Answer from the drawing. Dimensions are ordinates in mm from the lowest x, y and z of the part. Give positions to 0.01 mm unless a question says otherwise; leave off trailing zeros. Write each loop counter-clockwise with the first axis right and the second up, starting at its lowest first coordinate (ties: lowest second). Pieces come first, ordered by that corner, then holes. Notation, with made-up numbers: (51, 16) - (68, 16) arc R34 cw to (68, 54) - close; hole circle Ø3 at (-23.75, 83.25). An arc over 180 degrees is marked (long way). Answer as a JSON object with one key per item and string values. Group by question number.
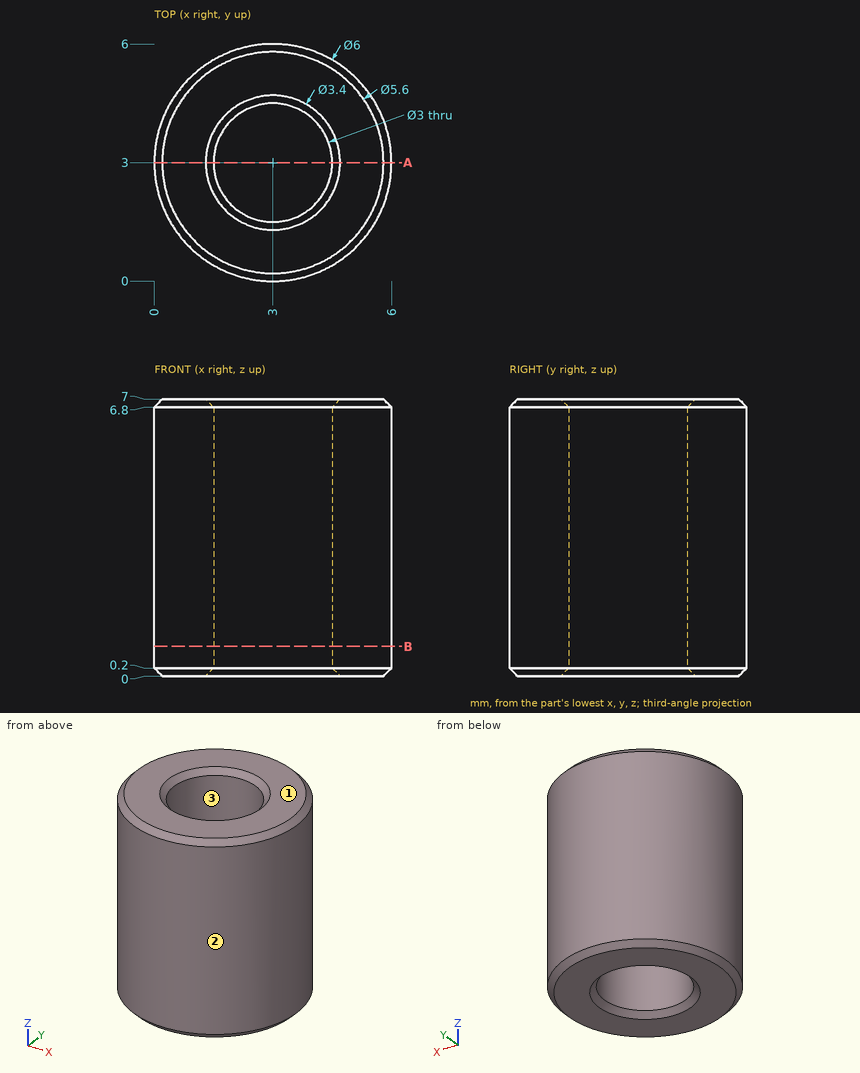
1) A flat-ended cylindrical pin translates along its axis: pin 1 Ø1 at (x, z) = (2.5, 2.5) entering from -Y. Find the tip coordinate at first contact, or state that the pin passes through.
2) Find section A-A, the plane y = 3. Write down the section's boundary in (x, z), and give its area (3 significant figures).
3) Find the intervals of material crossed by line 1 (Y direction, x = 3, z = 3.75); line 2 (Y direction, x = 4.1, z = 2.5); line 3 (X direction, y = 4, z = 6.25), in increasing order. Write a range as [from, to].
4) Find section B-B, the plane z = 0.75. Write down the section's boundary in (x, y), and give its area (3 significant figures).
5) For a pull along X with two mould halves and no side action, classify the marked faces 1, 2 and 3 as released by +X, released by -X, zero draft, split by the parting line, or undercut.
Values follow:
{
 "1": {"pin 1": "stops at y = 0"},
 "2": {"outline": "(0, 0.2) - (0.2, 0) - (1.3, 0) - (1.5, 0.2) - (1.5, 6.8) - (1.3, 7) - (0.2, 7) - (0, 6.8) - close; (4.5, 0.2) - (4.7, 0) - (5.8, 0) - (6, 0.2) - (6, 6.8) - (5.8, 7) - (4.7, 7) - (4.5, 6.8) - close", "area": "20.8 mm2"},
 "3": {"line 1": "y = [0, 1.5], [4.5, 6]", "line 2": "y = [0.21, 1.98], [4.02, 5.79]", "line 3": "x = [0.17, 1.88], [4.12, 5.83]"},
 "4": {"outline": "circle Ø6 at (3, 3); hole circle Ø3 at (3, 3)", "area": "21.2 mm2"},
 "5": {"face 1": "zero draft", "face 2": "split by the parting line", "face 3": "undercut"}
}
